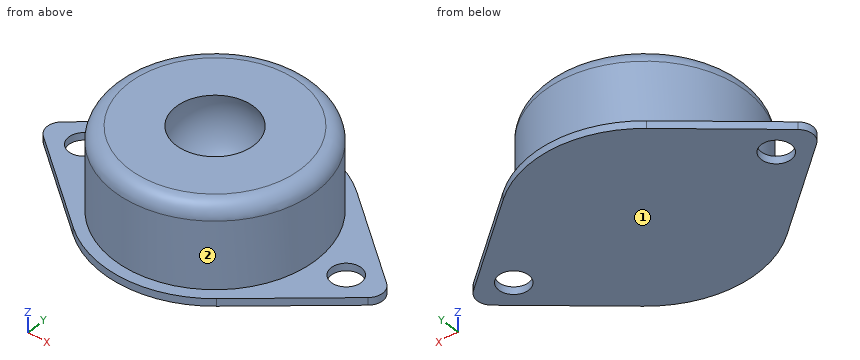
from build123d import *

# Parameters (mm, degrees)
SKETCH_1_R      = 13.5
SKETCH_1_R_2    = 2
EXTRUDE_3_DEPTH = 1
SKETCH_3_R      = 13.5
EXTRUDE_4_DEPTH = 12
FILLET_3_R      = 2


with BuildPart() as part:
    # 草图1 → 凸台-拉伸3 (new body)
    with BuildSketch(Plane.XY):
        with BuildLine():
            Line((-21.643262411, 1.539578937), (-9.574468085, 11.546842031))
            ThreePointArc((-9.574468085, 11.546842031), (0, 15), (9.574468085, 11.546842031))
            Line((9.574468085, 11.546842031), (21.643262411, 1.539578937))
            ThreePointArc((21.643262411, 1.539578937), (22.366666667, 0), (21.643262411, -1.539578937))
            Line((21.643262411, -1.539578937), (9.574468085, -11.546842031))
            ThreePointArc((9.574468085, -11.546842031), (0, -15), (-9.574468085, -11.546842031))
            Line((-9.574468085, -11.546842031), (-21.643262411, -1.539578937))
            ThreePointArc((-21.643262411, -1.539578937), (-22.366666667, 0), (-21.643262411, 1.539578937))
        make_face()
        Circle(SKETCH_1_R, mode=Mode.SUBTRACT)
        with Locations((-17.5, 0)):
            Circle(SKETCH_1_R_2, mode=Mode.SUBTRACT)
        with Locations((17.5, 0)):
            Circle(SKETCH_1_R_2, mode=Mode.SUBTRACT)
    extrude(amount=EXTRUDE_3_DEPTH)

    # 草图3 → 凸台-拉伸4 (add)
    with BuildSketch(Plane.XY):
        Circle(SKETCH_3_R)
    extrude(amount=EXTRUDE_4_DEPTH)

    # 圆角3
    fillet_3_edges = [part.edges().sort_by_distance(p)[0] for p in [
        (-13.5, 0, 12),
    ]]
    fillet(fillet_3_edges, radius=FILLET_3_R)

    # 草图4 → 切除-旋转9 (revolve, cut)
    with BuildSketch(Plane(origin=(0, 0, 0), x_dir=(1, 0, 0), z_dir=(0, 1, 0))):
        with BuildLine():
            Line((0, -12), (5.196152423, -12))
            ThreePointArc((5.196152423, -12), (5.196152423, -6), (0, -3))
            Line((0, -3), (0, -12))
        make_face()
    revolve(axis=Axis((0, 0, 0), (0, 0, 1)), mode=Mode.SUBTRACT)


solid = part.part
Could you check a few things on this model? Use its own coordinates, in mm. Face numbers are marked on the shaded views. A direction names the side the tool comes from. Give positions to 0.01 mm unless a question says otherwise; leave off trailing zeros. Loops run counter-clockwise (first coordinate to the right, second up) from the corner with the lowest first, then second, coordinate; pieces in that order, holes last. Notation, with made-up numbers: M 14.5,31.5 L 36.5,31.5 A8 cw 36.5,45.5 Z; hole C 14.5,-26 d4. An arc over 180 degrees is marked long. Answer as a JSON object with one key per item and string values.
Q1. Suppose I cut it at C-C, the plane z = 7.25. List the corners of the cut face in (x, y) for me, plus the area to 3 significant figures.
Values found:
{"outline": "C 0,0 d27; hole C 0,0 d11.48", "area": "469 mm²"}
Q2. If I drill on probe 1 along Z at (x, y) = (17, -4); probe 2 along X at (y, z) = (9.5, 10.25); probe 3 along Z at (x, y) = (-7, 9.25), over which ranges is the centre line in solid material (lowest first)? Write a range as [from, to].
Values found:
{"probe 1": "z = [0, 1]", "probe 2": "x = [-9.57, 9.57]", "probe 3": "z = [0, 12]"}
Q3. Suppose I cut it at A-A, the plane x = -17.5. List the corners of the cut face in (y, z) for me.
Values found:
{"outline": "M -4.98,0 L -2,0 L -2,1 L -4.98,1 Z; M 2,0 L 4.98,0 L 4.98,1 L 2,1 Z"}
Q4. Suppose I cut it at D-D, the plane z = 11. List the corners of the cut face in (x, y) for me, plus the area to 3 significant figures.
Values found:
{"outline": "C 0,0 d26.46; hole C 0,0 d11.31", "area": "450 mm²"}
Q5. For P1, Ø2, axis at x = 12.5, y = -5, coming from the +Z side; P2, Ø5, axis at y = -0.5, z = 5.5, coming from the -X side; P3, Ø1.5, axis at y = -2, z = 6, coming from the +X side, each with a flat end and sliding along its axis, tell me the tip position at first contact or that it passes through.
Values found:
{"P1": "stops at z = 11.75", "P2": "stops at x = -13.5", "P3": "stops at x = 13.44"}
Q6. For the marked faces 1 and 2, which set-ups out of +Z, -Z, +X, -X, +Y, -Y let a thin tool reach every point of the face, with its end or its side?
Values found:
{"face 1": "-Z, +X, -X, +Y, -Y", "face 2": "+Z"}
Q7. Suppose I cut it at B-B, the plane x = 0. List the corners of the cut face in (y, z) for me.
Values found:
{"outline": "M -15,0 L 15,0 L 15,1 L 13.5,1 L 13.5,10 A2 ccw 11.5,12 L 5.2,12 A6 cw long -5.2,12 L -11.5,12 A2 ccw -13.5,10 L -13.5,1 L -15,1 Z"}
